from build123d import *

# Parameters (mm, degrees)
SKETCH_1_R          = 1
EXTRUDE_1_DEPTH     = 5
EXTRUDE_1_2_DEPTH   = 5
EXTRUDE_1_3_DEPTH   = 5
SKETCH_2_W          = 12
SKETCH_2_H          = 10
EXTRUDE_6_DEPTH     = 2
SKETCH_1_6_R        = 2.1
CUT_EXTRUDE_2_DEPTH = 7
FILLET_1_R          = 5


with BuildPart() as part:
    # Sketch 1 → Extrude 1 (new body)
    with BuildSketch(Plane(origin=(0, 0, 0), x_dir=(1, 0, 0), z_dir=(0, 1, 0))):
        with Locations(Location((-5, 0, 0), (0, 0, 270))):
            Circle(SKETCH_1_R)
    extrude(amount=EXTRUDE_1_DEPTH)



with BuildPart() as body_2:
    # Sketch 1 → Extrude 1 2 (new body)
    with BuildSketch(Plane(origin=(0, 0, 0), x_dir=(1, 0, 0), z_dir=(0, 1, 0))):
        with Locations(Location((0, 5, 0), (0, 0, 270))):
            Circle(SKETCH_1_R)
    extrude(amount=EXTRUDE_1_2_DEPTH)


with BuildPart() as body_3:
    # Sketch 1 → Extrude 1 3 (new body)
    with BuildSketch(Plane(origin=(0, 0, 0), x_dir=(1, 0, 0), z_dir=(0, 1, 0))):
        with Locations(Location((5, 0, 0), (0, 0, 270))):
            Circle(SKETCH_1_R)
    extrude(amount=EXTRUDE_1_3_DEPTH)


with BuildPart() as part_1:
    add(part.part)

    add(body_2.part)  # Extrude 6 merges body 2

    add(body_3.part)  # Extrude 6 merges body 3
    # Sketch 2 → Extrude 6 (add)
    with BuildSketch(Plane(origin=(0, 5, 0), x_dir=(1, 0, 0), z_dir=(0, 1, 0))):
        with Locations((0, 1)):
            Rectangle(SKETCH_2_W, SKETCH_2_H)
    extrude(amount=EXTRUDE_6_DEPTH)

    # Sketch 1_6 → Cut-Extrude 2 (cut)
    with BuildSketch(Plane(origin=(0, 0, 0), x_dir=(1, 0, 0), z_dir=(0, 1, 0))):
        with Locations(Location((0, 0, 0), (0, 0, 90))):
            Circle(SKETCH_1_6_R)
    extrude(amount=CUT_EXTRUDE_2_DEPTH, mode=Mode.SUBTRACT)

    # Fillet 1
    fillet_1_edges = [part_1.edges().sort_by_distance(p)[0] for p in [
        (-6, 6, -6),
        (6, 6, -6),
    ]]
    fillet(fillet_1_edges, radius=FILLET_1_R)


solid = part_1.part
Work out the finished part from the listing and answer in its coordinate system (mm). A direction names the side the tool comes from. Coordinates: 2 decimals unless noted, no trailing zeros. Write each loop counter-clockwise with the first axis right and the second up, starting at its lowest first coordinate (ties: lowest second). Pieces come first, ordered by that corner, then holes. Notation, with made-up numbers: (81.25, -39) - (92.25, -39) arc R31 cw to (92.25, -9) - close; hole circle Ø5 at (89.25, 4). An arc over 180 degrees is marked (long way). One line per question, with ' | ' between items.
1) Find section A-A, the plane z = -1.5. Determine the outline of the cut face in (x, y), and give its area (3 significant figures).
Checks:
outline: (-5.97, 5) - (-1.47, 5) - (-1.47, 7) - (-5.97, 7) - close; (1.47, 5) - (5.97, 5) - (5.97, 7) - (1.47, 7) - close | area: 18.0 mm2
2) Find section C-C, the plane z = -5. Determine the outline of the cut face in (x, y).
Checks:
outline: (-4, 5) - (-1, 5) - (-1, 0) - (1, 0) - (1, 5) - (4, 5) - (4, 7) - (-4, 7) - close
3) Find section B-B, the plane y = 6. Determine the outline of the cut face in (x, z).
Checks:
outline: (-6, -1) arc R5 ccw to (-1, -6) - (1, -6) arc R5 ccw to (6, -1) - (6, 4) - (-6, 4) - close; hole circle Ø4.2 at (0, 0)
4) The mould has two halves that part along Z. Classify faces 3 (the face through (-0.631, 5.986, -2.003)), 4 (the face through (-0.6, 2.5, -5.8)), 5 (the face through (5, 0, 0)): +Z half, -Z half, draft (parallel to the pull), parting line (faces both ways), or undercut.
Checks:
face 3: undercut | face 4: parting line | face 5: draft
5) Flat-ended cylindrical pins translate along their axes: P1, Ø1.5, axis at x = -0.5, y = 3, coming from the +Z side; P2, Ø3, axis at x = 3, z = -2.5, coming from the -Y side. Find the tip coordinate at first contact, or state that the pin passes through.
Checks:
P1: z = -4 | P2: y = 5
6) Find section D-D, the plane x = 5. Determine the outline of the cut face in (y, z), and give its area (3 significant figures).
Checks:
outline: (0, -1) - (5, -1) - (5, -4) - (7, -4) - (7, 4) - (5, 4) - (5, 1) - (0, 1) - close | area: 26.0 mm2
7) Consider probe 1 along X at (y, z) = (6.1, 0); probe 2 along Y at (x, z) = (-3.5, -1.25); probe 3 along X at (y, z) = (3, 0.75). Determine where each line is inside the solid, lowest interval first. Write a range as [from, to].
Checks:
probe 1: [-6, -2.1], [2.1, 6] | probe 2: [5, 7] | probe 3: [-5.66, -4.34], [4.34, 5.66]
8) For faces 1 (the face through (-6, 6, 2)), 2 (the face through (1.2, 5, -2.2)), determine the directions among +Z, -Z, +X, -X, +Y, -Y from which every point of the face is accessible in a straight line to the end or side of a thin tool.
Checks:
face 1: +Z, -Z, -X, +Y, -Y | face 2: -Y
